Geometry check sheet. Reference: the model listing, model coordinates, mm. Face numbers are marked on the shaded views. Give positions to 0.01 mm unless a question says otherwise; leave off trailing zeros. Order: outer loops, then holes, each group sorted by start corner. A loop starts at its lowest first (then second) coordinate and runs counter-clockwise, first axis right, second up.
from build123d import *

# Parameters (mm, degrees)
F1_DEPTH = 60
F4_ANGLE = -180


with BuildPart() as f1:
    # F0 (on Top) → F1 (new body)
    with BuildSketch(Plane.XY):
        with BuildLine():
            ThreePointArc((23.366643, 7.5), (20.796862, 8.210918), (18.957842, 10.141509))
            ThreePointArc((18.957842, 10.141509), (-21.5, 0), (18.957842, -10.141509))
            ThreePointArc((18.957842, -10.141509), (20.796862, -8.210918), (23.366643, -7.5))
            Line((23.366643, -7.5), (26, -7.5))
            ThreePointArc((26, -7.5), (33.5, 0), (26, 7.5))
            Line((26, 7.5), (23.366643, 7.5))
        make_face()
        with BuildLine():
            ThreePointArc((17.959955, -8.8), (-20, 0), (17.959955, 8.8))
            ThreePointArc((17.959955, 8.8), (19.804193, 6.757359), (22.449944, 6))
            Line((22.449944, 6), (26, 6))
            ThreePointArc((26, 6), (32, 0), (26, -6))
            Line((26, -6), (22.449944, -6))
            ThreePointArc((22.449944, -6), (19.804193, -6.757359), (17.959955, -8.8))
        make_face(mode=Mode.SUBTRACT)
    extrude(amount=F1_DEPTH)

    # F3 (on offset) → F4 (revolve)
    with BuildSketch(Plane.XY.offset(60)):
        with BuildLine():
            ThreePointArc((17.959955, -8.8), (-4.516685, -19.483315), (-20, 0))
            Line((-20, 0), (-21.5, 0))
            ThreePointArc((-21.5, 0), (-5.227638, -20.854779), (18.957842, -10.141509))
            ThreePointArc((18.957842, -10.141509), (20.796862, -8.210918), (23.366643, -7.5))
            Line((23.366643, -7.5), (26, -7.5))
            ThreePointArc((26, -7.5), (31.303301, -5.303301), (33.5, 0))
            Line((33.5, 0), (32, 0))
            ThreePointArc((32, 0), (30.242641, -4.242641), (26, -6))
            Line((26, -6), (22.449944, -6))
            ThreePointArc((22.449944, -6), (19.804193, -6.757359), (17.959955, -8.8))
        make_face()
    revolve(axis=Axis((6, 0, 60), (1, 0, 0)), revolution_arc=F4_ANGLE)


solid = f1.part
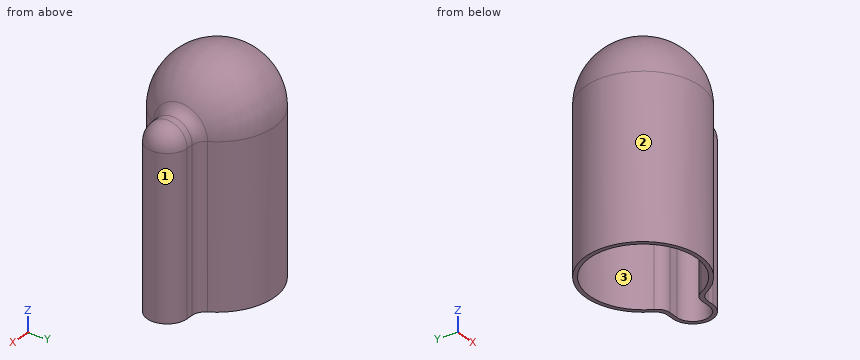
Item 1: Sectioned sample at A-A (z = 33). Enter the section's corners in (x, y), and give its area (3 significant figures).
Reported:
outline: (18.96, -10.14) arc R5 cw to (23.37, -7.5) - (26, -7.5) arc R7.5 ccw to (26, 7.5) - (23.37, 7.5) arc R5 cw to (18.96, 10.14) arc R21.5 ccw (long way) to start; hole (17.96, -8.8) arc R5 cw to (22.45, -6) - (26, -6) arc R6 ccw to (26, 6) - (22.45, 6) arc R5 cw to (17.96, 8.8) arc R20 ccw (long way) to start
area: 225 mm2
Item 2: Scan lines: L1, parallel to Y at x = 0, z = 19; L2, parallel to Y at x = 24, z = 59; L3, parallel to X at y = 0, z = 57.5. Record each from-to range of solid material in increasing order.
Reported:
L1: y = -21.5 to -20, 20 to 21.5
L2: y = -7.5 to -6, 6 to 7.5
L3: x = -21.5 to -20, 32 to 33.5
Item 3: Gauge pin test, flat ends, axial feed: pin 1 (10 mm diameter, centred on x = -4.5, y = -5, fed in from -Z); pin 2 (1.8 mm diameter, centred on x = 24, z = 31, fed in from +Y); pin 3 (12 mm diameter, centred on x = -3, y = 0.5, fed in from +Z). Record the tip position at first contact, or that the pin passes through.
Reported:
pin 1: stops at z = 76.2
pin 2: stops at y = 7.51
pin 3: stops at z = 81.5
Item 4: Sectioned sample at B-B (x = 25). Enter the section's corners in (y, z).
Reported:
outline: (-7.5, 0) - (-6, 0) - (-6, 60) arc R6 cw to (6, 60) - (6, 0) - (7.5, 0) - (7.5, 60) arc R7.5 ccw to (-7.5, 60) - close
Item 5: Draft check along X on the marked faces 1, 2 and 3. Enter one of: released by +X, released by -X, zero draft, split by the parting line, or undercut.
Reported:
face 1: released by +X
face 2: split by the parting line
face 3: undercut
